The listing builds one solid part. Answer for the finished solid, in the listing's coordinates (mm). A direction names the side the tool comes from. Round coordinates to 2 decimals unless told otherwise and drop trailing zeros. Order: outer loops, then holes, each group sorted by start corner. A loop starts at its lowest first (then second) coordinate and runs counter-clockwise, first axis right, second up. Notation, with made-up numbers: M 2.5,9 L 34.5,9 A25 ccw 34.5,30 Z; hole C -5,13.5 d7. An arc over 180 degrees is marked long. Put each result on its own line as item: value. Start each with the question number.
1. The mould has two halves that part along X. Classify faces 1 (the face through (-20, -13, 0)), 2 (the face through (-8.859, -8.797, -0.042)), 3 (the face through (-22, 12, 0)): +X half, -X half, draft (parallel to the pull), parting line (faces both ways), or undercut.
2. The part is cut by section B-B (x = -19). Give the vertices of the cut face in (y, z), then the cut area to 3 significant figures.
3. Which of the six approach directions +Z, -Z, +X, -X, +Y, -Y give full straight-line access (tool end or side, diameter ignored) to faces 4 (the face through (20, 14, 0)), 5 (the face through (-11, 0, -3)), 6 (the face through (8.797, 8.859, -0.042)), 7 (the face through (-20, 14, 0))?
4. The part is cut by section A-A (y = -2.5). Give the vertices of the cut face in (x, z), then the cut area to 3 significant figures.
5. The part is cut by section C-C (y = 13.5). Give the vertices of the cut face in (x, z), then the cut area to 3 significant figures.
6. The part is cut by section D-D (z = 2.5). Count the separate pieces of the cut face and the enclosed holes in it, then the cut area to 3 significant figures.
7. Each of these flat-tipped pins is pushed along its axis until it touches: pin 1 Ø2.5 at (y, z) = (-13.5, 0) entering from +X; pin 2 Ø5 at (x, y) = (5, -13.5) entering from +Z; pin 3 Ø2.5 at (y, z) = (13.5, 0) entering from -X. Where does it stop, or does it pass through?
8. Consider line 1 (Y direction, x = -22, z = 0); line 2 (Y direction, x = 5, z = 1.7); line 3 (X direction, y = -7, z = 0.5). Determine where each line is inside the solid, lowest interval first.
from build123d import *

# Parameters (mm, degrees)
SKETCH_1_W                = 50
SKETCH_1_H                = 34
EXTRUDE_1_DEPTH           = 6
SKETCH_2_W                = 20
SKETCH_2_H                = 20
CUT_EXTRUDE_1_DEPTH       = 31.822070015
HOLE_WIZARD_5_1_5_1_1_D   = 5.1
HOLE_WIZARD_3_0_3_1_D     = 3
HOLE_WIZARD_3_0_3_1_DEPTH = 5
HOLE_WIZARD_3_0_3_2_D     = 3
HOLE_WIZARD_3_0_3_2_DEPTH = 5
FILLET_1_R                = 4
CUT_EXTRUDE_3_REACH       = 32.822
SKETCH_9_R                = 1.55


with BuildPart() as part:
    # Sketch 1 → Extrude 1 (new body)
    with BuildSketch(Plane(origin=(0, 0, -3), x_dir=(-1, 0, 0), z_dir=(0, 0, -1))):
        Rectangle(SKETCH_1_W, SKETCH_1_H)
    extrude(amount=-EXTRUDE_1_DEPTH)

    # Sketch 2 → Cut-Extrude 1 (cut, through all)
    with BuildSketch(Plane.XY.offset(3)):
        Rectangle(SKETCH_2_W, SKETCH_2_H)
    extrude(amount=-CUT_EXTRUDE_1_DEPTH, mode=Mode.SUBTRACT)

    # Hole Wizard 5.1 _5.1_ _1 (through all)
    with Locations(Plane(origin=(0, 0, -3), x_dir=(-1, 0, 0), z_dir=(0, 0, -1))):
        with Locations((-19, 6), (19, -6), (-19, -6), (19, 6)):
            Hole(HOLE_WIZARD_5_1_5_1_1_D / 2)

    # Hole Wizard 3.0 _3_ _1
    with Locations(Plane.ZY.offset(25)):
        with Locations((0, -13.5), (0, 13.5)):
            Hole(HOLE_WIZARD_3_0_3_1_D / 2, depth=HOLE_WIZARD_3_0_3_1_DEPTH)

    # Hole Wizard 3.0 _3_ _2
    with Locations(Plane(origin=(25, 0, 0), x_dir=(0, 0, -1), z_dir=(1, 0, 0))):
        with Locations((0, -13.5), (0, 13.5)):
            Hole(HOLE_WIZARD_3_0_3_2_D / 2, depth=HOLE_WIZARD_3_0_3_2_DEPTH)

    # Fillet 1
    fillet_1_edges = [part.edges().sort_by_distance(p)[0] for p in [
        (10, 10, 0),
        (10, -10, 0),
        (-10, -10, 0),
        (-10, 10, 0),
    ]]
    fillet(fillet_1_edges, radius=FILLET_1_R)

    # Sketch 9 → Cut-Extrude 3 (cut, up to next)
    with BuildSketch(Plane.XY.offset(3), mode=Mode.PRIVATE) as cut_extrude_3_sk1:
        with Locations((5, -13.5)):
            Circle(SKETCH_9_R)
    cut_extrude_3_tool1 = extrude(cut_extrude_3_sk1.sketch, amount=-CUT_EXTRUDE_3_REACH, mode=Mode.PRIVATE) & part.part
    # Sketch 9 → Cut-Extrude 3 (cut, up to next)
    with BuildSketch(Plane.XY.offset(3), mode=Mode.PRIVATE) as cut_extrude_3_sk2:
        with Locations((-5, -13.5)):
            Circle(SKETCH_9_R)
    cut_extrude_3_tool2 = extrude(cut_extrude_3_sk2.sketch, amount=-CUT_EXTRUDE_3_REACH, mode=Mode.PRIVATE) & part.part
    cut_extrude_3_1 = cut_extrude_3_tool1.solids().sort_by_distance((5, -13.5, 3))[0]
    add(cut_extrude_3_1, mode=Mode.SUBTRACT)
    cut_extrude_3_2 = cut_extrude_3_tool2.solids().sort_by_distance((-5, -13.5, 3))[0]
    add(cut_extrude_3_2, mode=Mode.SUBTRACT)
    cut_extrude_3 = cut_extrude_3_1 + cut_extrude_3_2  # Cut-Extrude 3 as one shape, for the pattern or mirror that repeats it

    # Mirror 1: Cut-Extrude 3 across plane
    add(cut_extrude_3.mirror(Plane(origin=(0, 0, 0), x_dir=(0, 0, 1), z_dir=(0, -1, 0))), mode=Mode.SUBTRACT)


solid = part.part
Resolved:
1. face 1: -X half
1. face 2: undercut
1. face 3: draft
2. outline: M -17,-3 L -8.55,-3 L -8.55,3 L -17,3 Z; M -3.45,-3 L 3.45,-3 L 3.45,3 L -3.45,3 Z; M 8.55,-3 L 17,-3 L 17,3 L 8.55,3 Z
2. area: 143 mm2
3. face 4: +X
3. face 5: -Z, +X, -X, +Y, -Y
3. face 6: +Z, -Z
3. face 7: -X
4. outline: M -25,-3 L -10,-3 L -10,3 L -25,3 Z; M 10,-3 L 25,-3 L 25,3 L 10,3 Z
4. area: 180 mm2
5. outline: M -25,-3 L -6.55,-3 L -6.55,3 L -25,3 L -25,1.5 L -20,1.5 L -20,-1.5 L -25,-1.5 Z; M -3.45,-3 L 3.45,-3 L 3.45,3 L -3.45,3 Z; M 6.55,-3 L 25,-3 L 25,-1.5 L 20,-1.5 L 20,1.5 L 25,1.5 L 25,3 L 6.55,3 Z
5. area: 233 mm2
6. separate pieces: 1
6. enclosed holes: 9
6. area: 1,200 mm2
7. pin 1: x = 20
7. pin 2: z = 3
7. pin 3: x = -20
8. line 1: -17 to -15, -12 to 12, 15 to 17
8. line 2: -17 to -15.05, -11.95 to -10, 10 to 11.95, 15.05 to 17
8. line 3: -25 to -21.35, -16.65 to -9.87, 9.87 to 16.65, 21.35 to 25
